The listing builds one solid part. Answer for the finished solid, in the listing's coordinates (mm). A direction names the side the tool comes from. Give positions to 0.01 mm unless a question says otherwise; leave off trailing zeros. Write each loop counter-clockwise with the first axis right and the second up, starting at its lowest first coordinate (ties: lowest second). Pieces come first, ordered by that corner, then holes. Notation, with made-up numbers: (62.25, 62) - (100.25, 62) arc R28 ccw to (100.25, 85) - close; hole circle Ø10 at (68, 57.25). An arc over 180 degrees is marked (long way). Answer in a Markdown table with one row per item. Add a question column.
from build123d import *

# Parameters (mm, degrees)
BOSS_EXTRUDE1_DEPTH     = 101.6
SKETCH2_R               = 7.9375
SKETCH2_R_2             = 42.8625
CUT_EXTRUDE1_DEPTH      = 9.525
CUT_EXTRUDE1_DEPTH_BACK = 12.7
CUT_EXTRUDE2_REACH      = 14.7
SKETCH3_R               = 6.35


with BuildPart() as part:
    # Sketch1 → Boss-Extrude1 (new body, symmetric)
    with BuildSketch(Plane.XY):
        with BuildLine():
            Line((0, 0), (0, 101.6))
            Line((0, 101.6), (3.18008, 101.6))
            ThreePointArc((3.18008, 101.6), (9.911679988, 98.811679988), (12.7, 92.08008))
            Line((12.7, 92.08008), (12.7, 22.225))
            ThreePointArc((12.7, 22.225), (15.489807909, 15.489807909), (22.225, 12.7))
            Line((22.225, 12.7), (92.08008, 12.7))
            ThreePointArc((92.08008, 12.7), (98.811679988, 9.911679988), (101.6, 3.18008))
            Line((101.6, 3.18008), (101.6, 0))
            Line((101.6, 0), (0, 0))
        make_face()
    extrude(amount=BOSS_EXTRUDE1_DEPTH, both=True)

    # Sketch2 → Cut-Extrude1 (cut, two sides)
    with BuildSketch(Plane(origin=(0, 12.7, 0), x_dir=(1, 0, 0), z_dir=(0, 1, 0))) as cut_extrude1_sk:
        with Locations((45.9994, 53.213)):
            Circle(SKETCH2_R)
        with Locations((45.9994, -53.213)):
            Circle(SKETCH2_R)
        with Locations((45.9994, 0)):
            Circle(SKETCH2_R_2)
    extrude(amount=CUT_EXTRUDE1_DEPTH, mode=Mode.SUBTRACT)
    extrude(cut_extrude1_sk.sketch, amount=-CUT_EXTRUDE1_DEPTH_BACK, mode=Mode.SUBTRACT)

    # Sketch3 → Cut-Extrude2 (cut, up to next)
    with BuildSketch(Plane(origin=(12.7, 0, 0), x_dir=(0, 0, -1), z_dir=(1, 0, 0)), mode=Mode.PRIVATE) as cut_extrude2_sk1:
        with Locations((52.4891, 88.9)):
            Circle(SKETCH3_R)
    cut_extrude2_tool1 = extrude(cut_extrude2_sk1.sketch, amount=-CUT_EXTRUDE2_REACH, mode=Mode.PRIVATE) & part.part
    add(cut_extrude2_tool1.solids().sort_by_distance((12.7, 88.9, -52.4891))[0], mode=Mode.SUBTRACT)
    # Sketch3 → Cut-Extrude2 (cut, up to next)
    with BuildSketch(Plane(origin=(12.7, 0, 0), x_dir=(0, 0, -1), z_dir=(1, 0, 0)), mode=Mode.PRIVATE) as cut_extrude2_sk2:
        with Locations((-52.4891, 88.9)):
            Circle(SKETCH3_R)
    cut_extrude2_tool2 = extrude(cut_extrude2_sk2.sketch, amount=-CUT_EXTRUDE2_REACH, mode=Mode.PRIVATE) & part.part
    add(cut_extrude2_tool2.solids().sort_by_distance((12.7, 88.9, 52.4891))[0], mode=Mode.SUBTRACT)


solid = part.part
1. Section C-C (x = 50) is taken. Give the vertices of the cut face in (y, z), and give its area (3 significant figures).
2. Straight lines are drawn through the part: L1, parallel to Z at x = 4.5, y = 88.9; L2, parallel to Z at x = 5, y = 88 (3 decimals); L3, parallel to X at y = 59, z = -21.5. For each, find the intervals that lie inside material, in ascending order. Write a range as [from, to].
3. Section D-D (z = 0) is taken. Give the vertices of the cut face in (x, y) (3 decimals), and give its area (3 significant figures).
4. Given pin 1 Ø6 at (y, z) = (38, -61.5) entering from -X; pin 2 Ø3 at (x, z) = (6.5, -1.5) entering from -Y (3 decimals); pin 3 Ø3 at (y, z) = (83, -8.5) entering from +X; pin 4 Ø11.5 at (y, z) = (88.9, 52.49) entering from -X, each flat-ended and moving along its own axis, determine where each tip first touches the part or whether it passes through.
5. Section B-B (z = 87.5) is taken. Give the vertices of the cut face in (x, y) (3 decimals).
6. Section A-A (y = 88.9) is taken. Give the vertices of the cut face in (x, z).
7. The mould has two halves that part along Z. Classify faces 6 (the face through (15.42, 15.56, -63.77)), 7 (the face through (6.439, 94.254, -55.903)), 8 (the face through (28, 10, 101.6)): +Z half, -Z half, draft (parallel to the pull), parting line (faces both ways), or undercut.
8. A tool of negligible diameter and unlimited length cuts with its end or side. For faces 1 (the face through (28, 10, -101.6)), 2 (the face through (88, 12.7, -21)), 3 (the face through (9, 22.225, 0)), 4 (the face through (44.966, 6.439, -61.083)), 5 (the face through (3.18, 8.8, -1.88)), from which of +Z, -Z, +X, -X, +Y, -Y can it reach the whole face along a straight path? Write none if from no direction.
Geometry check:
| question | item | result |
|---|---|---|
| 1 | outline | (0, -101.6) - (12.7, -101.6) - (12.7, -60.07) - (0, -60.07) - close; (0, -46.36) - (12.7, -46.36) - (12.7, -42.68) - (0, -42.68) - close; (0, 42.68) - (12.7, 42.68) - (12.7, 46.36) - (0, 46.36) - close; (0, 60.07) - (12.7, 60.07) - (12.7, 101.6) - (0, 101.6) - close |
| 1 | area | 1,150 mm² |
| 2 | L1 | [-101.6, -58.84], [-46.14, 46.14], [58.84, 101.6] |
| 2 | L2 | [-101.6, -58.775], [-46.203, 46.203], [58.775, 101.6] |
| 2 | L3 | [0, 12.7] |
| 3 | outline | (0, 0) - (3.137, 0) - (3.137, 22.225) - (12.7, 22.225) - (12.7, 92.08) arc R9.52 ccw to (3.18, 101.6) - (0, 101.6) - close; (88.862, 0) - (101.6, 0) - (101.6, 3.18) arc R9.52 ccw to (92.08, 12.7) - (88.862, 12.7) - close |
| 3 | area | 1,200 mm² |
| 4 | pin 1 | x = 0 |
| 4 | pin 2 | y = 22.225 |
| 4 | pin 3 | x = 12.7 |
| 4 | pin 4 | through |
| 5 | outline | (0, 0) - (101.6, 0) - (101.6, 3.18) arc R9.52 ccw to (92.08, 12.7) - (22.225, 12.7) arc R9.525 cw to (12.7, 22.225) - (12.7, 92.08) arc R9.52 ccw to (3.18, 101.6) - (0, 101.6) - close |
| 6 | outline | (0, -101.6) - (12.7, -101.6) - (12.7, -58.84) - (0, -58.84) - close; (0, -46.14) - (12.7, -46.14) - (12.7, 46.14) - (0, 46.14) - close; (0, 58.84) - (12.7, 58.84) - (12.7, 101.6) - (0, 101.6) - close |
| 7 | face 6 | draft |
| 7 | face 7 | undercut |
| 7 | face 8 | +Z half |
| 8 | face 1 | -Z, +X, -X, +Y, -Y |
| 8 | face 2 | +Z, -Z, +X, +Y |
| 8 | face 3 | +X, -Y |
| 8 | face 4 | +Y, -Y |
| 8 | face 5 | -Y |
